Here's how the part is built. I have some questions about the finished solid (model axes, mm). A direction names the side the tool comes from. Round coordinates to 2 decimals unless told otherwise and drop trailing zeros. Write each loop counter-clockwise with the first axis right and the second up, starting at its lowest first coordinate (ties: lowest second). Pieces come first, ordered by that corner, then holes. Notation, with made-up numbers: (87.25, -33.5) - (124.25, -33.5) arc R21 cw to (124.25, -29.5) - close; hole circle Ø2 at (65, 44.5). An arc over 180 degrees is marked (long way). Write item = value, one per line. Start each with the question number.
Item 1: If we section it at A-A (y = -185): Please give me the cut outline in (x, z), and give its area (3 significant figures).
Item 2: If we section it at D-D (y = -10): Please give me the cut outline in (x, z), and give its area (3 significant figures).
Item 3: If I drill on line 1 along Y through (x, z) = (10, 1.8); line 2 along Y through (x, z) = (108, 3.1), over which ranges is the centre line in solid material (lowest first)? Write a range as [from, to].
Item 4: If we section it at B-B (x = 10): Please give me the cut outline in (y, z), and give its area (3 significant figures).
Item 5: Which directions (+Z, -Z, +X, -X, +Y, -Y) give clear straight access to the entire face, cutting with the end or side of a thin tool? Please do faces 4 (the face through (120, -175, 3)), 5 (the face through (240, -96, 2)).
Item 6: For P1, Ø2.5, axis at x = 118.5, z = 2, coming from the -Y side, with a flat end and sliding along its axis, tell me the tip position at first contact or that it passes through.
Item 7: Thinking about a two-plate mould opening in X: for faces 1 (the face through (118, -94, 5)), 2 (the face through (145, -183, 3)), 3 (the face through (0, -96, 2)), which applies, pulls with the +X half, pulls with the -X half, needs draft (parallel to the pull), parting line crosses it, or undercut?
Item 8: If we section it at C-C (z = 2.65): Please give me the cut outline in (x, y), and give its area (3 significant figures).
```python
from build123d import *

# Parameters (mm, degrees)
ESQUISSE1_W             = 240
ESQUISSE1_H             = 190
BOSS_EXTRU_1_DEPTH      = 5
ESQUISSE2_W             = 50
ESQUISSE2_H             = 15
ENL_V_MAT_EXTRU_1_DEPTH = 5
ESQUISSE3_R             = 3
ENL_V_MAT_EXTRU_2_DEPTH = 10


with BuildPart() as part:
    # Esquisse1 → Boss.-Extru.1 (new body)
    with BuildSketch(Plane.XY):
        with Locations((120, -95)):
            Rectangle(ESQUISSE1_W, ESQUISSE1_H)
    extrude(amount=BOSS_EXTRU_1_DEPTH)

    # Esquisse2 → Enlèv. mat.-Extru.1 (cut)
    with BuildSketch(Plane.XY.offset(5)):
        with Locations((120, -182.5)):
            Rectangle(ESQUISSE2_W, ESQUISSE2_H)
    extrude(amount=-ENL_V_MAT_EXTRU_1_DEPTH, mode=Mode.SUBTRACT)

    # Esquisse3 → Enlèv. mat.-Extru.2 (cut)
    with BuildSketch(Plane.XY.offset(5)):
        with Locations((10, -10)):
            Circle(ESQUISSE3_R)
        with Locations((10, -185)):
            Circle(ESQUISSE3_R)
        with Locations((230, -185)):
            Circle(ESQUISSE3_R)
        with Locations((230, -10)):
            Circle(ESQUISSE3_R)
    extrude(amount=-ENL_V_MAT_EXTRU_2_DEPTH, mode=Mode.SUBTRACT)


solid = part.part
```
Reply:
q1.outline = (0, 0) - (7, 0) - (7, 5) - (0, 5) - close; (13, 0) - (95, 0) - (95, 5) - (13, 5) - close; (145, 0) - (227, 0) - (227, 5) - (145, 5) - close; (233, 0) - (240, 0) - (240, 5) - (233, 5) - close
q1.area = 890 mm2
q2.outline = (0, 0) - (7, 0) - (7, 5) - (0, 5) - close; (13, 0) - (227, 0) - (227, 5) - (13, 5) - close; (233, 0) - (240, 0) - (240, 5) - (233, 5) - close
q2.area = 1,140 mm2
q3.line_1 = [-190, -188], [-182, -13], [-7, 0]
q3.line_2 = [-175, 0]
q4.outline = (-190, 0) - (-188, 0) - (-188, 5) - (-190, 5) - close; (-182, 0) - (-13, 0) - (-13, 5) - (-182, 5) - close; (-7, 0) - (0, 0) - (0, 5) - (-7, 5) - close
q4.area = 890 mm2
q5.face_4 = +Z, -Z, -Y
q5.face_5 = +Z, -Z, +X, +Y, -Y
q6.P1 = -175
q7.face_1 = needs draft
q7.face_2 = undercut
q7.face_3 = pulls with the -X half
q8.outline = (0, -190) - (95, -190) - (95, -175) - (145, -175) - (145, -190) - (240, -190) - (240, 0) - (0, 0) - close; hole circle Ø6 at (10, -185); hole circle Ø6 at (10, -10); hole circle Ø6 at (230, -185); hole circle Ø6 at (230, -10)
q8.area = 44,700 mm2
